Geometry check sheet. Reference: the model listing, model coordinates, mm. A direction names the side the tool comes from. Round coordinates to 2 decimals unless told otherwise and drop trailing zeros. Write each loop counter-clockwise with the first axis right and the second up, starting at its lowest first coordinate (ties: lowest second). Pieces come first, ordered by that corner, then holes. Notation, with made-up numbers: M -25.75,-37.5 L 4.25,-37.5 A37 cw 4.25,0.5 Z; hole C 4,29.5 d1. An arc over 180 degrees is marked long. Use a Markdown table: item, result.
```python
from build123d import *

# Parameters (mm, degrees)
SKETCH1_R           = 7
BOSS_EXTRUDE1_DEPTH = 34
SKETCH2_R           = 7.5
BOSS_EXTRUDE2_DEPTH = 2
SKETCH3_R           = 6
BOSS_EXTRUDE3_DEPTH = 19
SKETCH4_R           = 4
CUT_EXTRUDE1_DEPTH  = 21.5
CUT_EXTRUDE2_REACH  = 15.5
SKETCH6_W           = 5
SKETCH6_H           = 4.6
CUT_EXTRUDE3_DEPTH  = 19


with BuildPart() as part:
    # Sketch1 → Boss-Extrude1 (new body)
    with BuildSketch(Plane.XY):
        Circle(SKETCH1_R)
    extrude(amount=BOSS_EXTRUDE1_DEPTH)

    # Sketch2 → Boss-Extrude2 (add)
    with BuildSketch(Plane.XY.offset(34)):
        Circle(SKETCH2_R)
    extrude(amount=BOSS_EXTRUDE2_DEPTH)

    # Sketch3 → Boss-Extrude3 (add)
    with BuildSketch(Plane.XY.offset(36)):
        Circle(SKETCH3_R)
    extrude(amount=BOSS_EXTRUDE3_DEPTH)

    # Sketch4 → Cut-Extrude1 (cut)
    with BuildSketch(Plane.XY.offset(55)):
        Circle(SKETCH4_R)
    extrude(amount=-CUT_EXTRUDE1_DEPTH, mode=Mode.SUBTRACT)

    # Sketch5 → Cut-Extrude2 (cut, up to next)
    with BuildSketch(Plane(origin=(0, 6, 0), x_dir=(1, 0, 0), z_dir=(0, 1, 0)), mode=Mode.PRIVATE) as cut_extrude2_sk1:
        with BuildLine():
            Line((-1.5, -47.5), (-1.5, -36.5))
            ThreePointArc((-1.5, -36.5), (0, -35), (1.5, -36.5))
            Line((1.5, -36.5), (1.5, -47.5))
            ThreePointArc((1.5, -47.5), (0, -49), (-1.5, -47.5))
        make_face()
    cut_extrude2_tool1 = extrude(cut_extrude2_sk1.sketch, amount=-CUT_EXTRUDE2_REACH, mode=Mode.PRIVATE) & part.part
    add(cut_extrude2_tool1.solids().sort_by_distance((0, 6, 42))[0], mode=Mode.SUBTRACT)

    # Sketch6 → Cut-Extrude3 (cut)
    with BuildSketch(Plane(origin=(0, 0, 31.9), x_dir=(-1, 0, 0), z_dir=(0, 0, -1))):
        with Locations((0, 7)):
            Rectangle(SKETCH6_W, SKETCH6_H)
    extrude(amount=CUT_EXTRUDE3_DEPTH, mode=Mode.SUBTRACT)


solid = part.part
```
Item 1: Access from +Z, -Z, +X, -X, +Y, -Y to the whole of each face (thin tool, end or side, straight path). Record for faces 5 (the face through (-1.517, -6.834, 16.762)), 6 (the face through (0, 5, 35)), 7 (the face through (0, 6, 12.9)), 8 (the face through (-1.42, -3.92, 55)), 9 (the face through (-1.301, -5.857, 45.367)).
Outcome:
| item | result |
|---|---|
| face 5 | -Z |
| face 6 | none |
| face 7 | +Y |
| face 8 | +Z, +X, -X, +Y, -Y |
| face 9 | +Z |
Item 2: Cross-section at D-D, the plane x = 4.5. Record the cut outline in (y, z), and give its area (3 significant figures).
Outcome:
| item | result |
|---|---|
| outline | M -6,34 L -5.36,34 L -5.36,0 L 5.36,0 L 5.36,34 L 6,34 L 6,36 L 3.97,36 L 3.97,55 L -3.97,55 L -3.97,36 L -6,36 Z |
| area | 539 mm2 |
Item 3: Material ranges on line 1 along Z through (x, y) = (-1.25, 4.75); line 2 along Z through (x, y) = (2.25, -6.5); line 3 along Y through (x, z) = (0, 40.25), recorded low to high. Write a range as from..to.
Outcome:
| item | result |
|---|---|
| line 1 | z = 0..12.9, 31.9..35.67, 48.33..55 |
| line 2 | z = 0..36 |
| line 3 | y = -6..-4 |
Item 4: Cross-section at C-C, the plane z = 9. Record the cut outline in (x, y), and give its area (3 significant figures).
Outcome:
| item | result |
|---|---|
| outline | C 0,0 d14 |
| area | 154 mm2 |
Item 5: Cross-section at B-B, the plane y = 0. Record the cut outline in (x, z), and give its area (3 significant figures).
Outcome:
| item | result |
|---|---|
| outline | M -7.5,34 L -7,34 L -7,0 L 7,0 L 7,34 L 7.5,34 L 7.5,36 L 6,36 L 6,55 L 4,55 L 4,33.5 L -4,33.5 L -4,55 L -6,55 L -6,36 L -7.5,36 Z |
| area | 562 mm2 |
Item 6: Go/stop test with flat-tipped pins: pin 1 (0.8 mm diameter, centred on x = 0.5, z = 35.5, fed in from -Y); pin 2 (1.7 mm diameter, centred on y = 4.5, z = 44.5, fed in from -X); pin 3 (5 mm diameter, centred on x = -2, z = 26.5, fed in from -Y); pin 4 (4 mm diameter, centred on x = 2, z = 7, fed in from +Y). Record where each tip stops, or that it passes through.
Outcome:
| item | result |
|---|---|
| pin 1 | stops at y = -7.5 |
| pin 2 | stops at x = -4.76 |
| pin 3 | stops at y = -7 |
| pin 4 | stops at y = 7 |
Item 7: Cross-section at A-A, the plane x = 0. Record the cut outline in (y, z), and give its area (3 significant figures).
Outcome:
| item | result |
|---|---|
| outline | M -7.5,34 L -7,34 L -7,0 L 7,0 L 7,12.9 L 4.7,12.9 L 4.7,31.9 L 7,31.9 L 7,34 L 7.5,34 L 7.5,36 L 6,36 L 6,35 L 4,35 L 4,33.5 L -4,33.5 L -4,55 L -6,55 L -6,36 L -7.5,36 Z; M 4,49 L 6,49 L 6,55 L 4,55 Z |
| area | 490 mm2 |
Item 8: Mould release check, pull along Y, two halves, no side actions. Record for faces 1 (the face through (-0.867, -3.905, 44.4)), 2 (the face through (-1.5, 5, 42)), 3 (the face through (0, 6, 35.6)), 4 (the face through (0, 4.7, 23)): +Y half, -Y half, draft (parallel to the pull), parting line (faces both ways), or undercut.
Outcome:
| item | result |
|---|---|
| face 1 | undercut |
| face 2 | draft |
| face 3 | undercut |
| face 4 | +Y half |
